Design review of the part shown in the three views and the two pictorial views. Dimensions are in mm from the part's minimum x, y and z. Coordinates: 2 decimals unless noted, no trailing zeros. Order: outer loops, then holes, each group sorted by start corner. A loop starts at its lowest first (then second) coordinate and runs counter-clockwise, first axis right, second up. Notation, with made-up numbers: (71.25, 83.25) - (78.25, 83.25) arc R24 cw to (78.25, 121.25) - close; hole circle Ø3 at (-0.75, 6). An arc over 180 degrees is marked (long way). One line per item, written item: value. Start each with the question number.
(1) Consider section C-C on x = 61. Write out the cut boundary in (y, z).
(2) Mouldability with a two-part tool opening along Z and no side actions: class the marked faces 1 and 2 as released by +Z, released by -Z, zero draft, split by the parting line, or undercut.
(3) Consider section A-A on z = 13.5. Write out the cut boundary in (x, y).
(4) Consider section D-D on z = 30.5. Write out the cut boundary in (x, y).
(5) To check wall thickness, follow line 1 along Z through (x, y) = (58.5, 3.5); line 2 along X through (y, z) = (2, 45) (1 decimal); line 3 along Z through (x, y) = (52, 5) (1 decimal). State the ranges of each line that lie inside material, in increasing order.
(6) Consider section B-B on y = 1.25. Count the separate pieces of the cut face and the enclosed holes in it, then the cut area to 3 significant figures.
(7) Clearance check with flat-ended pins moving along their axes: pin 1 (1 mm diameter, centred on y = 5.5, z = 34, fed in from +X); pin 2 (2 mm diameter, centred on x = 30, y = 3.5, fed in from -Z); pin 3 (2 mm diameter, centred on x = 38, y = 3, fed in from -Z); pin 4 (4 mm diameter, centred on x = 5.67, z = 93.14, fed in from +Y). State where each tip first meets the part, or that it passes through.
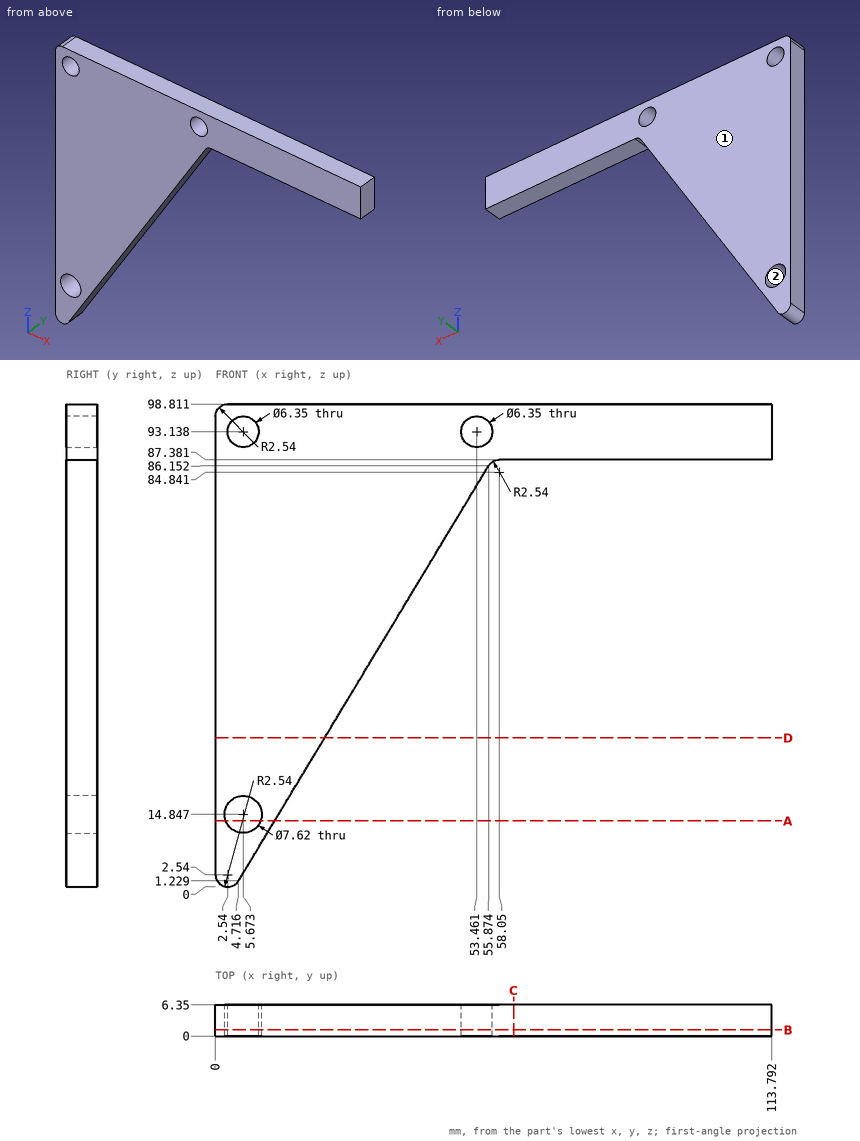
Geometry check:
1. outline: (0, 87.38) - (6.35, 87.38) - (6.35, 98.81) - (0, 98.81) - close
2. face 1: zero draft
2. face 2: undercut
3. outline: (0, 0) - (2.11, 0) - (2.11, 6.35) - (0, 6.35) - close; (9.24, 0) - (12.11, 0) - (12.11, 6.35) - (9.24, 6.35) - close
4. outline: (0, 0) - (22.35, 0) - (22.35, 6.35) - (0, 6.35) - close
5. line 1: z = 87.38 to 98.81
5. line 2: x = 0 to 31.1
5. line 3: z = 79.7 to 90.3, 96 to 98.8
6. separate pieces: 1
6. enclosed holes: 3
6. area: 3,840 mm^2
7. pin 1: stops at x = 24.76
7. pin 2: stops at z = 41.54
7. pin 3: stops at z = 54.82
7. pin 4: passes through
